Work out the finished part from the listing and answer in its coordinate system (mm). A direction names the side the tool comes from. Coordinates: 2 decimals unless noted, no trailing zeros. Write each loop counter-clockwise with the first axis right and the second up, starting at its lowest first coordinate (ties: lowest second). Pieces come first, ordered by that corner, then holes. Notation, with made-up numbers: (60.25, 37) - (67.25, 37) arc R8 cw to (67.25, 47) - close; hole circle Ø8 at (19.5, 59.25). An arc over 180 degrees is marked (long way). One line per item, written item: value.
```python
from build123d import *

# Parameters (mm, degrees)
SKETCH004_R      = 8.23
EXTRUDE004_DEPTH = 8
EXTRUDE005_DEPTH = 2
ARRAY_Z_COUNT    = 2
ARRAY_Z_PITCH    = 4


with BuildPart() as eixo1:
    # Sketch004 → Extrude004 (new body)
    with BuildSketch(Plane.XY):
        Circle(SKETCH004_R)
    extrude(amount=EXTRUDE004_DEPTH)


with BuildPart() as eixo_maior:
    # Sketch005 (on Face8 of Extrude002) → Extrude005 (new body)
    with BuildSketch(Plane.XY.offset(2)):
        with BuildLine():
            Line((-4, 16), (4, 16))
            Line((4, 6.9282032303), (4, 16))
            ThreePointArc((4, -6.9282032303), (8, 0), (4, 6.9282032303))
            Line((4, -6.9282032303), (4, -16))
            Line((4, -16), (-4, -16))
            Line((-4, -6.9282032303), (-4, -16))
            ThreePointArc((-4, 6.9282032303), (-8, 0), (-4, -6.9282032303))
            Line((-4, 16), (-4, 6.9282032303))
        make_face()
    extrude(amount=EXTRUDE005_DEPTH)

    # Array Z: Eixo Maior ×2


with BuildPart() as eixo_maior_1:
    add(eixo_maior.part)
    with Locations(*[(0, 0, i * ARRAY_Z_PITCH) for i in range(1, ARRAY_Z_COUNT)]):
        add(eixo_maior.part)

    # Fusion001: union Eixo1
    add(eixo1.part)


solid = eixo_maior_1.part
```
Item 1: Determine the mould class of faces 6 (the face through (0, -12, 2)), 7 (the face through (4, 12, 3)), 8 (the face through (0, 12, 4)), 9 (the face through (0, 0, 8)) for opening direction Z: +Z half, -Z half, draft (parallel to the pull), parting line (faces both ways), or undercut.
Evaluation:
face 6: -Z half
face 7: draft
face 8: undercut
face 9: +Z half
Item 2: Section C-C, the plane x = 0 is taken. Determine the outline of the cut face in (y, z).
Evaluation:
outline: (-16, 2) - (-8.23, 2) - (-8.23, 0) - (8.23, 0) - (8.23, 2) - (16, 2) - (16, 4) - (8.23, 4) - (8.23, 6) - (16, 6) - (16, 8) - (-16, 8) - (-16, 6) - (-8.23, 6) - (-8.23, 4) - (-16, 4) - close
Item 3: Which of the six approach directions +Z, -Z, +X, -X, +Y, -Y give full straight-line access (tool end or side, diameter ignored) to faces 1 (the face through (-4, 12, 7)), 2 (the face through (4, -12, 3)), 3 (the face through (-4, -12, 3)), 4 (the face through (4, 12, 7)), 5 (the face through (0, 16, 3))?
Evaluation:
face 1: +Z, -Z, -X, +Y
face 2: +Z, -Z, +X, -Y
face 3: +Z, -Z, -X, -Y
face 4: +Z, -Z, +X, +Y
face 5: +Z, -Z, +X, -X, +Y
Item 4: Given pin 1 (1.6 mm diameter, centred on y = -13.5, z = 7, fed in from -X); pin 2 (0.6 mm diameter, centred on y = -13.5, z = 2.5, fed in from +X); pin 3 (1.5 mm diameter, centred on y = 6, z = 3, fed in from +X); pin 4 (3 mm diameter, centred on y = -0.5, z = 6, fed in from -X), each flat-ended and moving along its own axis, determine where each tip first touches the part or whether it passes through.
Evaluation:
pin 1: stops at x = -4
pin 2: stops at x = 4
pin 3: stops at x = 6.34
pin 4: stops at x = -8.23
Item 5: Section A-A, the plane y = -14 is taken. Determine the outline of the cut face in (x, z), then the cut area to 3 significant figures.
Evaluation:
outline: (-4, 2) - (4, 2) - (4, 4) - (-4, 4) - close; (-4, 6) - (4, 6) - (4, 8) - (-4, 8) - close
area: 32.0 mm2
Item 6: Section B-B, the plane z = 2.5 is taken. Determine the outline of the cut face in (x, y).
Evaluation:
outline: (-4, -16) - (4, -16) - (4, -7.19) arc R8.23 ccw to (4, 7.19) - (4, 16) - (-4, 16) - (-4, 7.19) arc R8.23 ccw to (-4, -7.19) - close
Item 7: Section D-D, the plane x = 2.25 is taken. Determine the outline of the cut face in (y, z).
Evaluation:
outline: (-16, 2) - (-7.92, 2) - (-7.92, 0) - (7.92, 0) - (7.92, 2) - (16, 2) - (16, 4) - (7.92, 4) - (7.92, 6) - (16, 6) - (16, 8) - (-16, 8) - (-16, 6) - (-7.92, 6) - (-7.92, 4) - (-16, 4) - close
Item 8: Consider probe 1 along Z at (x, y) = (-1.75, 10); probe 2 along X at (y, z) = (13.5, 7.5); probe 3 along Y at (x, z) = (5.5, 7.5). Determine where each line is inside the solid, lowest interval first.
Evaluation:
probe 1: z = 2 to 4, 6 to 8
probe 2: x = -4 to 4
probe 3: y = -6.12 to 6.12
